Read the model definition and answer for the solid it produces. Units are mm, in the model's axes. A direction names the side the tool comes from. Round coordinates to 2 decimals unless told otherwise and drop trailing zeros. Loops run counter-clockwise (first coordinate to the right, second up) from the corner with the lowest first, then second, coordinate; pieces in that order, holes last. Notation, with made-up numbers: M 53.5,7 L 103.5,7 A21 cw 103.5,19 Z; hole C 68.5,45.5 d4. An arc over 180 degrees is marked long. Write each question's results on one line, items separated by ' | '.
```python
from build123d import *

# Parameters (mm, degrees)
ESQUISSE1_W                  = 40
ESQUISSE1_H                  = 34
BOSS_EXTRU_1_DEPTH           = 20
ESQUISSE2_W                  = 40
ESQUISSE2_H                  = 5
BOSS_EXTRU_3_DEPTH           = 20
ESQUISSE4_R                  = 4.5
ENL_V_MAT_EXTRU_1_DEPTH      = 21
ESQUISSE5_R                  = 8.1
ENL_V_MAT_EXTRU_2_DEPTH      = 12
ENL_V_MAT_EXTRU_3_DEPTH      = 21
ESQUISSE8_R                  = 2.2
ENL_V_MAT_EXTRU_5_DEPTH      = 6
ESQUISSE10_R                 = 4.5
BOSS_EXTRU_4_DEPTH           = 1
ESQUISSE11_W                 = 40
ESQUISSE11_H                 = 8
ENL_V_MAT_EXTRU_6_DEPTH      = 6
CONG_6_R                     = 4
ESQUISSE14_R                 = 1.65
ENL_V_MAT_EXTRU_7_DEPTH      = 6
ENL_V_MAT_EXTRU_7_DEPTH_BACK = 36


with BuildPart() as part:
    # Esquisse1 → Boss.-Extru.1 (new body)
    with BuildSketch(Plane.XY):
        Rectangle(ESQUISSE1_W, ESQUISSE1_H)
    extrude(amount=BOSS_EXTRU_1_DEPTH)

    # Esquisse2 → Boss.-Extru.3 (add)
    with BuildSketch(Plane.XY.offset(20)):
        with Locations((0, 14.5)):
            Rectangle(ESQUISSE2_W, ESQUISSE2_H)
    extrude(amount=BOSS_EXTRU_3_DEPTH)

    # Esquisse4 → Enlèv. mat.-Extru.1 (cut, through all)
    with BuildSketch(Plane.XY.offset(20)):
        with Locations((0, -3)):
            Circle(ESQUISSE4_R)
    extrude(amount=-ENL_V_MAT_EXTRU_1_DEPTH, mode=Mode.SUBTRACT)

    # Esquisse5 → Enlèv. mat.-Extru.2 (cut)
    with BuildSketch(Plane(origin=(0, 0, 0), x_dir=(-1, 0, 0), z_dir=(0, 0, -1))):
        with Locations((0, -3)):
            Circle(ESQUISSE5_R)
    extrude(amount=-ENL_V_MAT_EXTRU_2_DEPTH, mode=Mode.SUBTRACT)

    # Esquisse6 → Enlèv. mat.-Extru.3 (cut, through all)
    with BuildSketch(Plane.XY.offset(20)):
        Polygon((-20, -17), (-20, -2), (-15, -2), (-15, -7), (-15, -17), align=None)
        Polygon((20, 12), (15, 5), (15, -17), (20, -17), align=None)
    extrude(amount=-ENL_V_MAT_EXTRU_3_DEPTH, mode=Mode.SUBTRACT)

    # Esquisse8 → Enlèv. mat.-Extru.5 (cut, through all)
    with BuildSketch(Plane.XZ.offset(-12)):
        with Locations((-15, 26)):
            Circle(ESQUISSE8_R)
        with Locations((15, 26)):
            Circle(ESQUISSE8_R)
    extrude(amount=-ENL_V_MAT_EXTRU_5_DEPTH, mode=Mode.SUBTRACT)

    # Esquisse10 → Boss.-Extru.4 (add)
    with BuildSketch(Plane(origin=(0, 0, 12), x_dir=(-1, 0, 0), z_dir=(0, 0, -1))):
        with Locations((0, -3)):
            Circle(ESQUISSE10_R)
    extrude(amount=-BOSS_EXTRU_4_DEPTH)

    # Esquisse11 → Enlèv. mat.-Extru.6 (cut, through all)
    with BuildSketch(Plane.XZ.offset(-12)):
        with Locations((0, 36)):
            Rectangle(ESQUISSE11_W, ESQUISSE11_H)
    extrude(amount=-ENL_V_MAT_EXTRU_6_DEPTH, mode=Mode.SUBTRACT)

    # Congé6
    cong_6_edges = [part.edges().sort_by_distance(p)[0] for p in [
        (-20, 14.5, 32),
        (20, 14.5, 32),
    ]]
    fillet(cong_6_edges, radius=CONG_6_R)

    # Esquisse14 → Enlèv. mat.-Extru.7 (cut, two sides)
    with BuildSketch(Plane(origin=(15, 0, 0), x_dir=(0, 0, -1), z_dir=(1, 0, 0))) as enl_v_mat_extru_7_sk:
        with Locations((-5.5, -10.3)):
            Circle(ESQUISSE14_R)
        with Locations((-5.5, 4.9)):
            Circle(ESQUISSE14_R)
    extrude(amount=ENL_V_MAT_EXTRU_7_DEPTH, mode=Mode.SUBTRACT)
    extrude(enl_v_mat_extru_7_sk.sketch, amount=-ENL_V_MAT_EXTRU_7_DEPTH_BACK, mode=Mode.SUBTRACT)


solid = part.part
```
1. Find section C-C, the plane y = -10.3. Give the vertices of the cut face in (x, z).
Completed:
outline: M -15,0 L -3.51,0 L -3.51,3.85 L -15,3.85 Z; M -15,7.15 L -3.51,7.15 L -3.51,12 L 3.51,12 L 3.51,7.15 L 15,7.15 L 15,20 L -15,20 Z; M 3.51,0 L 15,0 L 15,3.85 L 3.51,3.85 Z
2. Determine the mould class of faces 6 (the face through (0, 17, 16)), 7 (the face through (8.09, -2.64, 5.92)), 8 (the face through (-18.859, 14.535, 30.797)) for opening direction Y: released by +Y, released by -Y, zero draft, split by the parting line, or undercut.
Completed:
face 6: released by +Y | face 7: undercut | face 8: zero draft
3. Which of the six approach directions +Z, -Z, +X, -X, +Y, -Y give full straight-line access (tool end or side, diameter ignored) to faces 1 (the face through (-18, -2, 10)), 2 (the face through (0, -3, 13)), 3 (the face through (-5, 4, 0)), 4 (the face through (0, 12, 26)), 5 (the face through (18.859, 14.535, 30.797))?
Completed:
face 1: +Z, -Z, -X, -Y | face 2: +Z | face 3: -Z, +X, -X, +Y, -Y | face 4: +Z, +X, -X, -Y | face 5: +Z, +X, +Y, -Y
4. Find section D-D, the plane x = -7. Give the vertices of the cut face in (y, z).
Completed:
outline: M -17,0 L -7.08,0 L -7.08,12 L 1.08,12 L 1.08,0 L 17,0 L 17,32 L 12,32 L 12,20 L -17,20 Z; hole C -10.3,5.5 d3.3; hole C 4.9,5.5 d3.3
5. Find section A-A, the plane z = 26. Give the vertices of the cut face in (x, y).
Completed:
outline: M -20,12 L -17.2,12 L -17.2,17 L -20,17 Z; M -12.8,12 L 12.8,12 L 12.8,17 L -12.8,17 Z; M 17.2,12 L 20,12 L 20,17 L 17.2,17 Z
6. Given P1, Ø3, axis at x = -4, y = -7, coming from the +Z side; P2, Ø1.5, axis at x = -16.5, z = 10.5, coming from the -Y side; P3, Ø12, axis at y = -7.5, z = 24.5, coming from the +X side; P4, Ø3, axis at y = 4.9, z = 5.5, coming from the -X side, each flat-ended and moving along its own axis, determine where each tip first touches the part or whether it passes through.
Completed:
P1: stops at z = 20 | P2: stops at y = -2 | P3: stops at x = 15 | P4: passes through
7. Find the intervals of material crossed by L1, parallel to Z at x = 15, y = 15.1; L2, parallel to Y at x = -16.5, z = 5.5; L3, parallel to Z at x = -5, y = 4.9, in increasing order.
Completed:
L1: z = 0 to 23.8, 28.2 to 32 | L2: y = -2 to 3.25, 6.55 to 17 | L3: z = 0 to 3.85, 7.15 to 20
8. Find section B-B, the plane z = 15. Give the vertices of the cut face in (x, y).
Completed:
outline: M -20,-2 L -15,-2 L -15,-17 L 15,-17 L 15,5 L 20,12 L 20,17 L -20,17 Z; hole C 0,-3 d9
